from build123d import *

# Parameters (mm, degrees)
SKETCH1_R           = 3.175
BOSS_EXTRUDE1_DEPTH = 6.35
SKETCH2_R           = 1.75
CUT_EXTRUDE1_DEPTH  = 7.35
CIRPATTERN1_COUNT   = 4
FILLET1_R           = 12.7


with BuildPart() as part:
    # Sketch1 → Boss-Extrude1 (new body)
    with BuildSketch(Plane(origin=(0, 0, 0), x_dir=(1, 0, 0), z_dir=(0, 1, 0))):
        with BuildLine():
            Line((13.748153285, -7.9375), (42.847508948, 42.464062476))
            ThreePointArc((42.847508948, 42.464062476), (23.210569318, 55.681011996), (0, 60.325))
            Line((0, 60.325), (0, 56.515))
            ThreePointArc((0, 56.515), (14.981702707, 45.890162758), (9.909464895, 28.23765625))
            Line((9.909464895, 28.23765625), (-9.909464895, 12.40234375))
            ThreePointArc((-9.909464895, 12.40234375), (-10.349453758, -12.037625676), (13.748153285, -7.9375))
        make_face()
        Circle(SKETCH1_R, mode=Mode.SUBTRACT)
    extrude(amount=BOSS_EXTRUDE1_DEPTH)

    # Sketch2 → Cut-Extrude1 (cut, through all)
    with BuildSketch(Plane(origin=(0, 6.35, 0), x_dir=(1, 0, 0), z_dir=(0, 1, 0))):
        with Locations((8, 0)):
            Circle(SKETCH2_R)
    cut_extrude1 = extrude(amount=-CUT_EXTRUDE1_DEPTH, mode=Mode.SUBTRACT)

    # CirPattern1: Cut-Extrude1 ×4 about axis
    cirpattern1_axis = Axis((0, 0, 0), (0, 1, 0))
    for i in range(1, CIRPATTERN1_COUNT):
        add(cut_extrude1.rotate(cirpattern1_axis, i * 360 / CIRPATTERN1_COUNT), mode=Mode.SUBTRACT)

    # Fillet1
    fillet1_edges = [part.edges().sort_by_distance(p)[0] for p in [
        (42.847508948, 3.175, -42.464062476),
    ]]
    fillet(fillet1_edges, radius=FILLET1_R)


solid = part.part
Can you work these out from the model? Positions are in its coordinate system, mm. A direction names the side the tool comes from. Coordinates: 2 decimals unless noted, no trailing zeros. Order: outer loops, then holes, each group sorted by start corner. A loop starts at its lowest first (then second) coordinate and runs counter-clockwise, first axis right, second up. Notation, with made-up numbers: (-29, 21.5) -> (23, 21.5) arc R26 cw to (23, 38.5) -> close; hole circle Ø2 at (62, 27.25). An arc over 180 degrees is marked (long way). Use one line per item in the form item = value.
Q1. Will these pins go through, and if not, where does the flat tip stop? P1, Ø1.5, axis at x = 12.5, y = 1, coming from the -Z side; P2, Ø2, axis at x = 4.5, y = 2.5, coming from the -Z side; P3, Ø1.5, axis at x = 1, y = 1.5, coming from the -Z side.
From the geometry:
P1 = -59.17
P2 = -60.22
P3 = -60.32
Q2. We'd pull the mould along Z, two halves only. Please class faces 1 (the face through (-9.669, 3.219, 0.526)), 2 (the face through (11, 6.35, -23)), 3 (the face through (38.91, 3.22, -42.31)): released by +Z, released by -Z, zero draft, split by the parting line, or undercut.
From the geometry:
face_1 = undercut
face_2 = zero draft
face_3 = split by the parting line
Q3. I need wall thicknesses on L1, parallel to X at y = 2.75, z = -8; L2, parallel to Z at x = 29, y = 1; L3, parallel to X at y = 5.75, z = -50.5. Which ranges of each line are inside material? Lowest first, please.
From the geometry:
L1 = -13.71 to -1.75, 1.75 to 22.95
L2 = -52.9 to -18.48
L3 = 12.44 to 33
Q4. Imagine slicing it at C-C, the plane z = -8. List the corners of the cut face in (x, y) for me, then the cut area to 3 significant figures.
From the geometry:
outline = (-13.71, 0) -> (-1.75, 0) -> (-1.75, 6.35) -> (-13.71, 6.35) -> close; (1.75, 0) -> (22.95, 0) -> (22.95, 6.35) -> (1.75, 6.35) -> close
area = 211 mm²
Q5. Which directions (+Z, -Z, +X, -X, +Y, -Y) give clear straight access to the entire face, cutting with the end or side of a thin tool? Please do faces 4 (the face through (0, 3, -58)), 5 (the face through (-10.64, 3.13, 11.78)), 6 (the face through (0.1, 3.1, -20.4)).
From the geometry:
face_4 = -Z, -X, +Y, -Y
face_5 = +Y, -Y
face_6 = -X, +Y, -Y
Q6. Imagine slicing it at B-B, the plane x = 5. List the corners of the cut face in (y, z) for me (3 decimals).
From the geometry:
outline = (0, -60.117) -> (6.35, -60.117) -> (6.35, -55.707) -> (0, -55.707) -> close; (0, -24.315) -> (6.35, -24.315) -> (6.35, 15.067) -> (0, 15.067) -> close
Q7. Imagine slicing it at A-A, the plane y = 3. Give the number of separate pieces and of enclosed holes in the cut face, then the cut area to 3 significant figures.
From the geometry:
separate_pieces = 1
enclosed_holes = 5
area = 1,940 mm²
Q8. Imagine slicing it at D-D, the plane z = 0. List the corners of the cut face in (x, y) for me (3 decimals).
From the geometry:
outline = (-15.875, 0) -> (-9.75, 0) -> (-9.75, 6.35) -> (-15.875, 6.35) -> close; (-6.25, 0) -> (-3.175, 0) -> (-3.175, 6.35) -> (-6.25, 6.35) -> close; (3.175, 0) -> (6.25, 0) -> (6.25, 6.35) -> (3.175, 6.35) -> close; (9.75, 0) -> (18.331, 0) -> (18.331, 6.35) -> (9.75, 6.35) -> close
